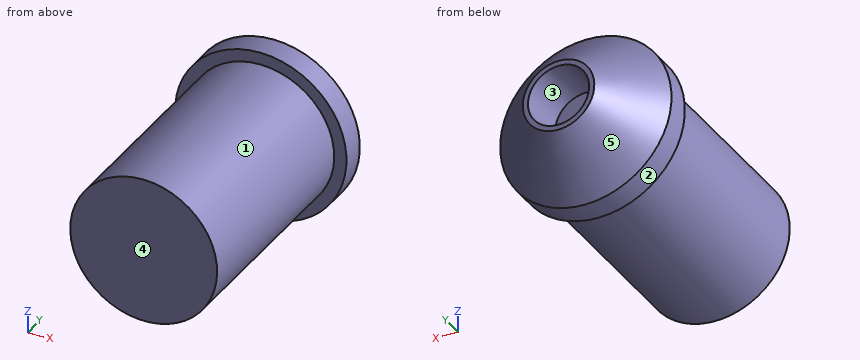
```python
from build123d import *

# Parameters (mm, degrees)
SKETCH2_R           = 3
BOSS_EXTRUDE1_DEPTH = 8.75
SKETCH5_R           = 3.5
BOSS_EXTRUDE4_DEPTH = 1


with BuildPart() as part:
    # Sketch2 → Boss-Extrude1 (new body)
    with BuildSketch(Plane(origin=(0, 0, 0), x_dir=(1, 0, 0), z_dir=(0, 1, 0))):
        with Locations(Location((0, 0, 0), (0, 0, 270))):
            Circle(SKETCH2_R)
    extrude(amount=-BOSS_EXTRUDE1_DEPTH)

    # Sketch5 → Boss-Extrude4 (add)
    with BuildSketch(Plane(origin=(0, 0, 0), x_dir=(1, 0, 0), z_dir=(0, 1, 0))):
        with Locations(Location((0, 0, 0), (0, 0, 270))):
            Circle(SKETCH5_R)
    extrude(amount=BOSS_EXTRUDE4_DEPTH)

    # Sketch6 → Revolve1 (revolve)
    with BuildSketch(Plane.XY, mode=Mode.PRIVATE) as revolve1_sk:
        Polygon((-3.5, 1), (-1.461129737, 3.038870263), (-1.25, 3.038870263), (-1.25, 1), align=None)
    revolve(revolve1_sk.sketch.rotate(Axis((0, 3.038870263, 0), (0, -1, 0)), 270), axis=Axis((0, 3.038870263, 0), (0, -1, 0)))


solid = part.part
```
The model under review builds one solid part; all positions refer to its coordinate system, in mm. Face numbers are marked on the shaded views. A direction names the side the tool comes from. Give positions to 0.01 mm unless a question says otherwise; leave off trailing zeros. Write each loop counter-clockwise with the first axis right and the second up, starting at its lowest first coordinate (ties: lowest second). Pieces come first, ordered by that corner, then holes.
(1) To check wall thickness, follow L1, parallel to X at y = 2.25, z = -1; L2, parallel to X at y = 1.7, z = 0; L3, parallel to Y at x = -0.5, z = 0.5. State the ranges of each line that lie inside material, in increasing order.
(2) Consider section B-B, the plane x = 0. Give the boundary of the cut face in (y, z).
(3) The part is to be moulded in two halves that separate along X. For the marked faces 3, 4 and 5, say which applies: released by +X, released by -X, zero draft, split by the parting line, or undercut.
(4) For P1, Ø1, axis at x = -1, z = -2, coming from the +Y side; P2, Ø1.5, axis at x = 1.5, y = -3, coming from the -Z side; P3, Ø2, axis at y = -2, z = 2, coming from the +X side, all flat-tipped, find the tip position at first contact; note any pin that passes through.
(5) Consider section D-D, the plane y = -4.75. Give the boundary of the cut face in (x, z).
(6) Consider section C-C, the plane y = 1.25. Give the boundary of the cut face in (x, z), and give its area (3 significant figures).
(7) Consider section A-A, the plane z = 0. Give the boundary of the cut face in (x, y).
(8) Tool access review of the marked faces 1 and 2: name each direction out of +Z, -Z, +X, -X, +Y, -Y from which nothing blocks a thin tool from reaching the whole face with its end or side.
Returned:
1. L1: x = -2.02 to -0.75, 0.75 to 2.02
1. L2: x = -2.8 to -1.25, 1.25 to 2.8
1. L3: y = -8.75 to 1
2. outline: (-8.75, -3) - (0, -3) - (0, -3.5) - (1, -3.5) - (3.04, -1.46) - (3.04, -1.25) - (1, -1.25) - (1, 1.25) - (3.04, 1.25) - (3.04, 1.46) - (1, 3.5) - (0, 3.5) - (0, 3) - (-8.75, 3) - close
3. face 3: undercut
3. face 4: zero draft
3. face 5: split by the parting line
4. P1: stops at y = 2.76
4. P2: stops at z = -2.9
4. P3: stops at x = 2.83
5. outline: circle Ø6 at (0, 0)
6. outline: circle Ø6.5 at (0, 0); hole circle Ø2.5 at (0, 0)
6. area: 28.3 mm2
7. outline: (-3.5, 0) - (-3, 0) - (-3, -8.75) - (3, -8.75) - (3, 0) - (3.5, 0) - (3.5, 1) - (1.46, 3.04) - (1.25, 3.04) - (1.25, 1) - (-1.25, 1) - (-1.25, 3.04) - (-1.46, 3.04) - (-3.5, 1) - close
8. face 1: -Y
8. face 2: +Y, -Y
